The listing builds one solid part. Answer for the finished solid, in the listing's coordinates (mm). Coordinates: 2 decimals unless noted, no trailing zeros. Write each loop counter-clockwise with the first axis right and the second up, starting at its lowest first coordinate (ties: lowest second). Pieces come first, ordered by that corner, then holes. Notation, with made-up numbers: M 87,58 L 93,58 A12 ccw 93,81 Z; hole C 5.5,76.25 d11. An arc over 180 degrees is marked long. Write item = value, one per line. Start each with the question number.
```python
from build123d import *

# Parameters (mm, degrees)
F0_R     = 11.0109
F1_DEPTH = 7


with BuildPart() as f1:
    # F0 (on Top) → F1 (new body)
    with BuildSketch(Plane.XY):
        with BuildLine():
            ThreePointArc((50.523907, -22.296429), (54.036916, -11.393316), (55.224957, 0))
            ThreePointArc((55.224957, 0), (54.036465, 11.395451), (50.522145, 22.300421))
            ThreePointArc((50.522145, 22.300421), (25.146702, 24.789823), (23.020236, 50.198253))
            ThreePointArc((23.020236, 50.198253), (0, 55.224957), (-23.020236, 50.198253))
            ThreePointArc((-23.020236, 50.198253), (-20.337253, 44.76174), (-19.414414, 38.769875))
            ThreePointArc((-19.414414, 38.769875), (-30.010396, 21.170629), (-50.522145, 22.300421))
            ThreePointArc((-50.522145, 22.300421), (-55.224957, 0), (-50.522145, -22.300421))
            ThreePointArc((-50.522145, -22.300421), (-30.010396, -21.170629), (-19.414414, -38.769875))
            ThreePointArc((-19.414414, -38.769875), (-20.337253, -44.76174), (-23.020236, -50.198253))
            ThreePointArc((-23.020236, -50.198253), (-0.002182, -55.224957), (23.016269, -50.200072))
            ThreePointArc((23.016269, -50.200072), (25.143646, -24.78681), (50.523907, -22.296429))
        make_face()
        with Locations((0, -42.291)):
            Circle(F0_R, mode=Mode.SUBTRACT)
        with Locations((-42.291, 0)):
            Circle(F0_R, mode=Mode.SUBTRACT)
        Circle(F0_R, mode=Mode.SUBTRACT)
        with Locations((0, 42.029381)):
            Circle(F0_R, mode=Mode.SUBTRACT)
        with Locations((42.037, 0)):
            Circle(F0_R, mode=Mode.SUBTRACT)
    extrude(amount=F1_DEPTH)


solid = f1.part
```
1. The part is cut by section D-D, the plane z = 4. Write down the section's boundary in (x, y).
2. The part is cut by section A-A, the plane x = 0. Write down the section's boundary in (y, z), and give its area (3 significant figures).
3. For a pull along X with two mould halves and no side action, classify faces 1 (the face through (25.42, 24.52, 3.45)), 2 (the face through (0.332, 55.224, 3.451)), 3 (the face through (54.07, 11.24, 3.45)) as pulls with the +X half, pulls with the -X half, needs draft (parallel to the pull), parting line crosses it, or undercut.
4. Each of these flat-tipped pins is pushed along its axis until it touches: pin 1 (1.5 mm diameter, centred on y = -30.5, z = 5, fed in from -X); pin 2 (1.5 mm diameter, centred on y = -31, z = 2, fed in from +X); pin 3 (13 mm diameter, centred on x = 42.037, y = 0, fed in from +Z); pin 4 (3 mm diameter, centred on y = 29, z = 5.5, fed in from -X). Where does it stop, or does it pass through?
5. The part is cut by section B-B, the plane y = 45. Write down the section's boundary in (x, z), and give its area (3 significant figures).
6. Straight lines are drawn through the part: L1, parallel to Y at x = 0, z = 2.5; L2, parallel to X at y = 9.5, z = 1.5; L3, parallel to Y at x = 3, z = 4.75. For each, find the intervals that lie inside material, in ascending order. Write a range as [from, to].
7. The part is cut by section C-C, the plane x = 40.5. Write down the section's boundary in (y, z), and give its area (3 significant figures).
Solution:
q1.outline = M -50.52,-22.3 A19.91 cw -19.41,-38.77 A19.91 cw -23.02,-50.2 A55.22 ccw 23.02,-50.2 A19.92 cw 50.52,-22.3 A55.22 ccw 55.22,0 A55.22 ccw 50.52,22.3 A19.91 cw 23.02,50.2 A55.22 ccw -23.02,50.2 A19.91 cw -19.41,38.77 A19.91 cw -50.52,22.3 A55.22 ccw Z; hole C -42.29,0 d22.02; hole C 0,-42.29 d22.02; hole C 0,0 d22.02; hole C 0,42.03 d22.02; hole C 42.04,0 d22.02
q2.outline = M -55.22,0 L -53.3,0 L -53.3,7 L -55.22,7 Z; M -31.28,0 L -11.01,0 L -11.01,7 L -31.28,7 Z; M 11.01,0 L 31.02,0 L 31.02,7 L 11.01,7 Z; M 53.04,0 L 55.22,0 L 55.22,7 L 53.04,7 Z
q2.area = 311 mm^2
q3.face_1 = undercut
q3.face_2 = parting line crosses it
q3.face_3 = pulls with the +X half
q4.pin_1 = -21.57
q4.pin_2 = 21.32
q4.pin_3 = through
q4.pin_4 = -22.91
q5.outline = M -20.41,0 L -10.6,0 L -10.6,7 L -20.41,7 Z; M 10.6,0 L 20.41,0 L 20.41,7 L 10.6,7 Z
q5.area = 137 mm^2
q6.L1 = [-55.22, -53.3], [-31.28, -11.01], [11.01, 31.02], [53.04, 55.22]
q6.L2 = [-54.4, -47.86], [-36.72, -5.57], [5.57, 36.47], [47.6, 54.4]
q6.L3 = [-55.14, -52.89], [-31.7, -10.59], [10.59, 31.44], [52.62, 55.14]
q7.outline = M -18.89,0 L -10.9,0 L -10.9,7 L -18.89,7 Z; M 10.9,0 L 18.89,0 L 18.89,7 L 10.9,7 Z
q7.area = 112 mm^2
